from build123d import *

# Parameters (mm, degrees)
ENL_V_MAT_EXTRU_1_DEPTH      = 34.496268449
ENL_V_MAT_EXTRU_1_DEPTH_BACK = 34.496268449
CONG_1_R                     = 2
CONG_2_R                     = 2
ENL_V_START                  = -5
ESQUISSE4_R                  = 6.7
ENL_V_MAT_EXTRU_2_DEPTH      = 5


with BuildPart() as part:
    # Esquisse2 → Révolution1 (revolve)
    with BuildSketch(Plane.XY, mode=Mode.PRIVATE) as r_volution1_sk:
        Polygon((4.7, 0), (4.7, 20), (6.7, 20), (6.7, 15), (19, 20), (19, 14), (9, 9.93495935), (6.7, 0), align=None)
    revolve(r_volution1_sk.sketch.rotate(Axis((0, 0, 0), (0, 1, 0)), 90), axis=Axis((0, 0, 0), (0, 1, 0)))

    # Esquisse3 → Enlèv. mat.-Extru.1 (cut, two sides: drawn at the far end of the back side and taken through both)
    with BuildSketch(Plane(origin=(0, 20, 0), x_dir=(1, 0, 0), z_dir=(0, 1, 0)).offset(-ENL_V_MAT_EXTRU_1_DEPTH_BACK)):
        with BuildLine():
            Line((-1.5, 9.583318841), (-2.474226804, 15.807536232))
            ThreePointArc((-2.474226804, 15.807536232), (-13.856406461, 8), (-14.92684135, -5.761024849))
            Line((-14.92684135, -5.761024849), (-9.049397568, -3.492621315))
            ThreePointArc((-9.049397568, -3.492621315), (-8.400446417, 4.85), (-1.5, 9.583318841))
        make_face()
        with BuildLine():
            Line((9.049397568, -3.492621315), (14.92684135, -5.761024849))
            ThreePointArc((14.92684135, -5.761024849), (13.856406461, 8), (2.474226804, 15.807536232))
            Line((2.474226804, 15.807536232), (1.5, 9.583318841))
            ThreePointArc((1.5, 9.583318841), (8.400446417, 4.85), (9.049397568, -3.492621315))
        make_face()
        with BuildLine():
            Line((-7.549397568, -6.090697526), (-12.452614546, -10.046511383))
            ThreePointArc((-12.452614546, -10.046511383), (0, -16), (12.452614546, -10.046511383))
            Line((12.452614546, -10.046511383), (7.549397568, -6.090697526))
            ThreePointArc((7.549397568, -6.090697526), (0, -9.7), (-7.549397568, -6.090697526))
        make_face()
    extrude(amount=ENL_V_MAT_EXTRU_1_DEPTH + ENL_V_MAT_EXTRU_1_DEPTH_BACK, mode=Mode.SUBTRACT)

    # Congé1
    cong_1_edges = [part.edges().sort_by_distance(p)[0] for p in [
        (0, 14, 19),
        (0, 20, 19),
    ]]
    fillet(cong_1_edges, radius=CONG_1_R)

    # Congé2
    cong_2_edges = [part.edges().sort_by_distance(p)[0] for p in [
        (-14.92684135, 15.780487805, 5.761024849),
        (-2.474226804, 15.780487805, -15.807536232),
        (-1.5, 13.219512195, -9.583318841),
        (-9.049397568, 13.219512195, 3.492621315),
        (2.474226804, 15.780487805, -15.807536232),
        (14.92684135, 15.780487805, 5.761024849),
        (9.049397568, 13.219512195, 3.492621315),
        (1.5, 13.219512195, -9.583318841),
        (12.452614546, 15.780487805, 10.046511383),
        (-12.452614546, 15.780487805, 10.046511383),
        (-7.549397568, 13.219512195, 6.090697526),
        (7.549397568, 13.219512195, 6.090697526),
    ]]
    fillet(cong_2_edges, radius=CONG_2_R)

    # Esquisse4 → Enlèv. mat.-Extru.2 (cut)
    with BuildSketch(Plane(origin=(0, 20, 0), x_dir=(1, 0, 0), z_dir=(0, 1, 0)).offset(ENL_V_START)):
        Circle(ESQUISSE4_R)
    extrude(amount=ENL_V_MAT_EXTRU_2_DEPTH, mode=Mode.SUBTRACT)


solid = part.part
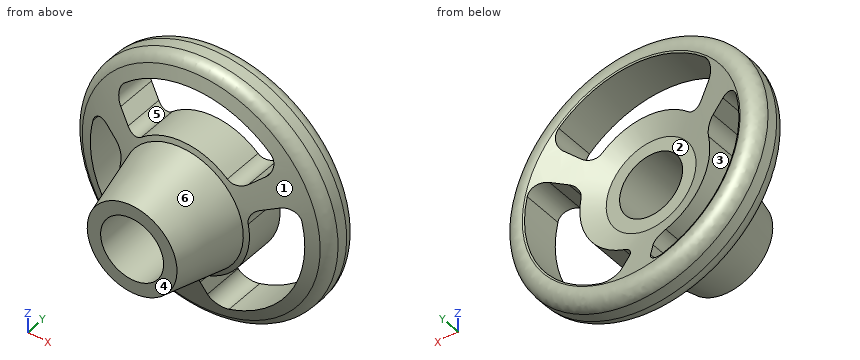
Read the model definition and answer for the solid it produces. Units are mm, in the model's axes. Face numbers are marked on the shaded views. A direction names the side the tool comes from. Round coordinates to 2 decimals unless told otherwise and drop trailing zeros. Write each loop counter-clockwise with the first axis right and the second up, starting at its lowest first coordinate (ties: lowest second). Pieces come first, ordered by that corner, then holes.
1. The part is cut by section A-A, the plane z = 0. State how many separate pieces and enclosed holes the cut face has, then the cut area to 3 significant figures.
2. The part is cut by section C-C, the plane y = 5.75. Determine the outline of the cut face in (x, z), then the cut area to 3 significant figures.
3. Given pin 1 Ø10 at (y, z) = (17, -13.5) entering from -X; pin 2 Ø4 at (y, z) = (7.5, -1) entering from +X; pin 3 Ø5 at (y, z) = (7, -11) entering from -X; pin 4 Ø1.5 at (x, z) = (-12.5, 12) entering from -Y, each flat-ended and moving along its own axis, determine where each tip first touches the part or whether it passes through.
4. Straight lines are drawn through the part: L1, parallel to Z at x = -7, y = 15; L2, parallel to X at y = 11, z = 0; L3, parallel to Y at x = -3.5, z = 5. For each, find the intervals that lie inside material, in ascending order.
5. Determine the mould class of the marked faces 4, 5 and 6 for opening direction Z: pulls with the +Z half, pulls with the -Z half, needs draft (parallel to the pull), parting line crosses it, or undercut.
6. Which of the six approach directions +Z, -Z, +X, -X, +Y, -Y give full straight-line access (tool end or side, diameter ignored) to the marked faces 1, 2 and 3?
Values:
1. separate pieces: 4
1. enclosed holes: 0
1. area: 148 mm2
2. outline: circle Ø16.06 at (0, 0); hole circle Ø9.4 at (0, 0)
2. area: 133 mm2
3. pin 1: stops at x = -16.99
3. pin 2: stops at x = 8.87
3. pin 3: passes through
3. pin 4: stops at y = 13.02
4. L1: z = -17.63 to -14.39, -6.71 to 6.93, 14.39 to 17.63
4. L2: x = -9.7 to -4.7, 4.7 to 9.7
4. L3: y = 0 to 15
5. face 4: needs draft
5. face 5: undercut
5. face 6: parting line crosses it
6. face 1: -Y
6. face 2: +Y
6. face 3: +Y, -Y
